Autodesk Inventor part; units mm, degrees
ref_plane "YZ Plane" through (0, 0, 0) normal (1, 0, 0) x (0, 1, 0)
ref_plane "XZ Plane" through (0, 0, 0) normal (0, 1, 0) x (-1, 0, 0)
ref_plane "XY Plane" through (0, 0, 0) normal (0, 0, 1) x (1, 0, 0)
sketch "Sketch1" plane through (0, 0, 0) normal (0, 0, 1) x (1, 0, 0)
  line L0 (-500, 1325) -> (500, 1325)
  line L1 (500, 1325) -> (500, -1325)
  line L2 (500, -1325) -> (-500, -1325)
  line L3 (-500, -1325) -> (-500, 1325)
  line L4 (-500, 1325) -> (500, -1325) construction
  line L5 (500, 1325) -> (-500, -1325) construction
  point P0 (0, 0)
  dimension "d0" = 1000
  dimension "d1" = 2650
extrude "Extrusion1" add sketch "Sketch1" along normal blind 100
sketch "Sketch2" plane through (-500, -1325, 0) normal (0, -1, 0) x (1, 0, 0)
  line L0 (0, 0) -> (1000, 0)
  line L1 (1000, 0) -> (1000, 100)
  line L2 (0, 100) -> (1000, 100)
  line L3 (0, 0) -> (0, 100)
  line L4 (0, 100) -> (1000, 100)
  line L5 (1000, 100) -> (977, 135)
  line L6 (977, 135) -> (937, 135)
  line L7 (937, 135) -> (914, 100)
  line L8 (687, 135) -> (664, 100)
  line L9 (727, 135) -> (687, 135)
  line L10 (750, 100) -> (727, 135)
  line L11 (437, 135) -> (414, 100)
  line L12 (477, 135) -> (437, 135)
  line L13 (500, 100) -> (477, 135)
  line L14 (187, 135) -> (164, 100)
  line L15 (227, 135) -> (187, 135)
  line L16 (250, 100) -> (227, 135)
  line L17 (-63, 135) -> (-86, 100)
  line L18 (-23, 135) -> (-63, 135)
  line L19 (0, 100) -> (-23, 135)
  line L20 (-90.1785, 102.7459) -> (-65.6973, 140)
  line L21 (-65.6973, 140) -> (-20.3027, 140)
  line L22 (-20.3027, 140) -> (5.983, 100)
  line L23 (-90.1785, 102.7459) -> (-86, 100)
  point P0 (500, 0)
  point P1 (5.983, 100)
  dimension "d4" = 86
  dimension "d5" = 40
  dimension "d6" = 35
  dimension "d11" = 250
  dimension "d16" = 5
  dimension "d17" = 5
extrude "Extrusion2" add sketch "Sketch2" against normal up to surface (2650 mm away) contours L19 L18 L17 L23 L20 L21 L22 L2 | L2 L7 L6 L5 | L14 L15 L16 L2 | L2 L8 L9 L10 | L11 L12 L13 L2
chamfer "Chamfer1" distance 10 angle 45 2 edges at (500, -1325, 50) (500, 1325, 50)
equation "\"d17\" = d16"
properties part number "Sandwich 5  roof long"
Geometry check sheet. Reference: the model listing, model coordinates, mm. A direction names the side the tool comes from. Give positions to 0.01 mm unless a question says otherwise; leave off trailing zeros. Loops run counter-clockwise (first coordinate to the right, second up) from the corner with the lowest first, then second, coordinate; pieces in that order, holes last. Notation, with made-up numbers: M 20.5,87.5 L 53.5,87.5 A15 cw 53.5,101.5 Z; hole C 28,38 d10. An arc over 180 degrees is marked long. Write item = value, one per line. Start each with the question number.
1. Tool access check on faces 5 (the face through (-169, 19, 100)), 6 (the face through (-58, 1325, 53)). Record the directions out of +Z, -Z, +X, -X, +Y, -Y that give a thin tool (end or side, any length) a straight path to the whole face; none if there is none.
2. Draft check along X on faces 1 (the face through (500, 18, 49)), 2 (the face through (-500, -19, 49)), 3 (the face through (-543, -19, 140)), 4 (the face through (-416, 19, 100)). Enter one of: +X half, -X half, draft (parallel to the pull), parting line (faces both ways), or undercut.
3. Section check B-B, the plane z = 44. Enter the section's corners in (x, y).
4. Go/stop test with flat-tipped pins: P1, Ø4, axis at x = 277.5, y = 245, coming from the -Z side; P2, Ø12, axis at x = -533, y = -615, coming from the -Z side; P3, Ø20, axis at x = -45.5, y = 86, coming from the +Z side; P4, Ø3, axis at y = -356, z = 19, coming from the -X side. Record where each tip stops, or that it passes through.
5. Thickness scan on probe 1 along X at (y, z) = (-666.5, 117); probe 2 along X at (y, z) = (886.5, 89); probe 3 along Z at (x, y) = (-52, 525.5). Record the ranges inside material, lowest first.
6. Section check A-A, the plane y = 819.5. Enter the section's corners in (x, z), plus the area to 3 significant figures.
7. Section check C-C, the plane x = 60. Enter the section's corners in (y, z), plus the area to 3 significant figures.
Values follow:
q1.face_5 = +Z, +Y, -Y
q1.face_6 = +Z, -Z, +X, -X, +Y
q2.face_1 = +X half
q2.face_2 = -X half
q2.face_3 = draft
q2.face_4 = undercut
q3.outline = M -500,-1325 L 490,-1325 L 500,-1315 L 500,1315 L 490,1325 L -500,1325 Z
q4.P1 = 0
q4.P2 = 135
q4.P3 = 135
q4.P4 = -500
q5.probe_1 = -580.81 to -574.83, -511.17 to -505.19, -324.83 to -261.17, -74.83 to -11.17, 175.17 to 238.83, 425.17 to 488.83
q5.probe_2 = -500 to 500
q5.probe_3 = 0 to 135
q6.outline = M -590.18,102.75 L -586,100 L -563,135 L -523,135 L -500,100 L -500,0 L 500,0 L 500,100 L 477,135 L 437,135 L 414,100 L 250,100 L 227,135 L 187,135 L 164,100 L 0,100 L -23,135 L -63,135 L -86,100 L -250,100 L -273,135 L -313,135 L -336,100 L -494.02,100 L -520.3,140 L -565.7,140 Z
q6.area = 109,000 mm^2
q7.outline = M -1325,0 L 1325,0 L 1325,100 L -1325,100 Z
q7.area = 265,000 mm^2
